Model file for the job. Use its own axes, mm. Coordinates: 2 decimals unless noted, no trailing zeros. Loops run counter-clockwise (first coordinate to the right, second up) from the corner with the lowest first, then second, coordinate; pieces in that order, holes last. Notation, with made-up numbers: M 19.25,42.25 L 61.25,42.25 A23 ccw 61.25,68.25 Z; hole C 75,-10.75 d9. An arc over 180 degrees is marked long. Write item = value, one per line. Start each with the question number.
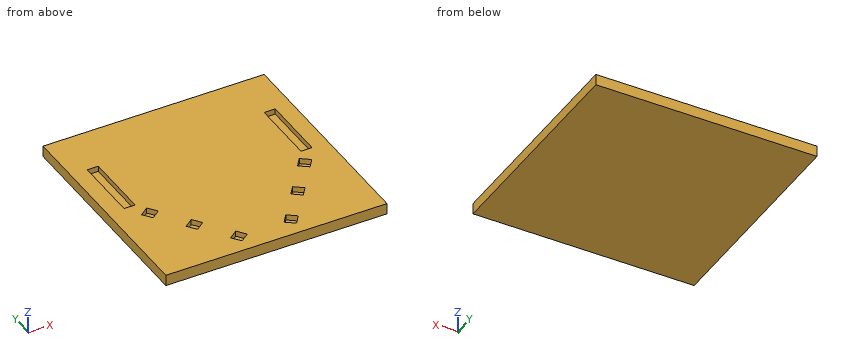
from build123d import *

# Parameters (mm, degrees)
F0_W     = 200
F0_H     = 200
F1_DEPTH = 10
F2_W     = 10
F2_H     = 60
F3_DEPTH = 5


with BuildPart() as f1:
    # F0 (on Top) → F1 (new body)
    with BuildSketch(Plane.XY):
        Rectangle(F0_W, F0_H)
    extrude(amount=F1_DEPTH)

    # F2 (on face) → F3 (cut)
    with BuildSketch(Plane.XY.offset(10)):
        with Locations((-80, 25)):
            Rectangle(F2_W, F2_H)
        with Locations((80, 25)):
            Rectangle(F2_W, F2_H)
        Polygon((-68.98185, -12.986355), (-76.968205, -19.004505), (-70.950055, -26.99086), (-62.9637, -20.97271), align=None)
        Polygon((-45.811971, -43.733822), (-53.798326, -49.751972), (-47.780176, -57.738328), (-39.793821, -51.720177), align=None)
        Polygon((-22.642093, -74.481289), (-30.628448, -80.49944), (-24.610298, -88.485795), (-16.623943, -82.467644), align=None)
        Polygon((22.642093, -74.481289), (16.623943, -82.467644), (24.610298, -88.485795), (30.628448, -80.49944), align=None)
        Polygon((76.968205, -19.004505), (68.98185, -12.986355), (62.9637, -20.97271), (70.950055, -26.99086), align=None)
        Polygon((47.780176, -57.738328), (53.798326, -49.751972), (45.811971, -43.733822), (39.793821, -51.720177), align=None)
    extrude(amount=-F3_DEPTH, mode=Mode.SUBTRACT)


solid = f1.part
Item 1: Cut at D-D (y = -46). Give the cut face in (x, z), plus the area to 3 significant figures.
Item 2: Probe L1, parallel to X at y = -18, z = 7; L2, parallel to X at y = 6, z = 8.75; L3, parallel to Y at x = -80, z = 6. List the from-to ranges inside material, lowest first.
Item 3: Cut at B-B (y = 8.5). Give the cut face in (x, z), plus the area to 3 significant figures.
Item 4: Pin check, flat tips, straight feed: pin 1 Ø15.5 at (x, y) = (-69.5, -20) entering from +Z; pin 2 Ø4 at (x, y) = (-23.5, -78.5) entering from +Z. Stop position of each tip, or through.
Item 5: Cut at A-A (z = 7.5). Give the number of separate pieces and of enclosed holes in the cut face, plus the area to 3 significant figures.
Item 6: Cut at C-C (x = -82). Give the cut face in (y, z), plus the area to 3 significant figures.
Reported:
q1.outline = M -100,0 L 100,0 L 100,10 L 48.82,10 L 48.82,5 L 44.1,5 L 44.1,10 L -44.1,10 L -44.1,5 L -48.82,5 L -48.82,10 L -100,10 Z
q1.area = 1,950 mm^2
q2.L1 = -100 to -75.64, -65.2 to 65.2, 75.64 to 100
q2.L2 = -100 to -85, -75 to 75, 85 to 100
q2.L3 = -100 to -5, 55 to 100
q3.outline = M -100,0 L 100,0 L 100,10 L 85,10 L 85,5 L 75,5 L 75,10 L -75,10 L -75,5 L -85,5 L -85,10 L -100,10 Z
q3.area = 1,900 mm^2
q4.pin_1 = 10
q4.pin_2 = 5
q5.separate_pieces = 1
q5.enclosed_holes = 8
q5.area = 38,200 mm^2
q6.outline = M -100,0 L 100,0 L 100,10 L 55,10 L 55,5 L -5,5 L -5,10 L -100,10 Z
q6.area = 1,700 mm^2
